Work out the finished part from the listing and answer in its coordinate system (mm). A direction names the side the tool comes from. Coordinates: 2 decimals unless noted, no trailing zeros. Loops run counter-clockwise (first coordinate to the right, second up) from the corner with the lowest first, then second, coordinate; pieces in that order, holes last. Notation, with made-up numbers: (73.5, 71) - (126.5, 71) arc R13 ccw to (126.5, 94) - close; hole circle Ø4 at (58, 68.25). An arc over 180 degrees is marked (long way). Write each question's results on one line, items separated by ' | '. Start each with the question number.
Item 1: Section D-D, the plane z = -2.4 is taken. Write down the section's boundary in (x, y).
Item 2: Consider probe 1 along X at (y, z) = (-5, 0); probe 2 along X at (y, z) = (-4.5, -0.35); probe 3 along Z at (x, y) = (-5, -3.5). Determine where each line is inside the solid, lowest interval first. Write a range as [from, to].
Item 3: Section B-B, the plane z = 0 is taken. Write down the section's boundary in (x, y).
Item 4: Section C-C, the plane y = -4.25 is taken. Write down the section's boundary in (x, z), plus the area to 3 significant figures.
Item 5: Each of these flat-tipped pins is pushed along its axis until it touches: pin 1 Ø1.9 at (x, z) = (5, 0) entering from +Y; pin 2 Ø1.1 at (x, z) = (-5, 0) entering from +Y. Where does it stop, or does it pass through?
Item 6: For a pull along X with two mould halves and no side action, classify faces 1 (the face through (-8, -4, 0)), 2 (the face through (-0.021, -1.318, -1.243)), 3 (the face through (4, -0.214, -1)), 4 (the face through (4.77, -3.954, 0.554)) as +X half, -X half, draft (parallel to the pull), parting line (faces both ways), or undercut.
Item 7: A tool of negligible diameter and unlimited length cuts with its end or side. For faces 5 (the face through (-0.021, -1.318, 1.757)), 6 (the face through (0.021, -1.318, 1.243)), 7 (the face through (0.021, -1.318, -1.757)), 8 (the face through (-5, -0.214, 1)), from which of +Z, -Z, +X, -X, +Y, -Y can it reach the whole face along a straight path? Write none if from no direction.
Item 8: Section A-A, the plane x = -5 is taken. Write down the section's boundary in (y, z).
from build123d import *

# Parameters (mm, degrees)
SKETCH_1_W               = 16
SKETCH_1_H               = 16
SKETCH_1_R               = 1.55
EXTRUDE_1_DEPTH          = 3
EXTRUDE_2_DEPTH          = 8
CUT_EXTRUDE_2_DEPTH      = 12.704699911
CUT_EXTRUDE_2_DEPTH_BACK = 12.704699911
SKETCH_8_R               = 0.6
CUT_EXTRUDE_3_DEPTH      = 12.704699911
CUT_EXTRUDE_START        = -0.2
SKETCH_10_W              = 16
SKETCH_10_H              = 6
SKETCH_10_R              = 0.6
CUT_EXTRUDE_7_DEPTH      = 0.2


with BuildPart() as part:
    # 草图1 → 凸台-拉伸1 (new, symmetric)
    with BuildSketch(Plane.XY):
        Rectangle(SKETCH_1_W, SKETCH_1_H)
        Circle(SKETCH_1_R, mode=Mode.SUBTRACT)
    extrude(amount=EXTRUDE_1_DEPTH, both=True)

    # 草图6 → 凸台-拉伸2 (add)
    with BuildSketch(Plane(origin=(0, 0, 0), x_dir=(1, 0, 0), z_dir=(0, 1, 0))):
        Polygon((-1.55, -1.743476048), (-1.55, -2.243476048), (1.55, -1.256523952), (1.55, -0.756523952), align=None)
        Polygon((-1.55, 1.256523952), (-1.55, 0.756523952), (1.55, 1.743476048), (1.55, 2.243476048), align=None)
    extrude(amount=-EXTRUDE_2_DEPTH)

    # 草图7 → 切除-拉伸2 (cut, two sides: drawn at the far end of the back side and taken through both)
    with BuildSketch(Plane.XY.offset(-CUT_EXTRUDE_2_DEPTH_BACK)):
        with BuildLine():
            Line((-8, -0.214092961), (-1.027941732, -0.214092961))
            ThreePointArc((-1.027941732, -0.214092961), (-0.107613153, 1.044470875), (1.05, 0))
            ThreePointArc((1.05, 0), (1.044470875, -0.107613153), (1.027941732, -0.214092961))
            Line((1.027941732, -0.214092961), (8, -0.214092961))
            Line((8, -0.214092961), (8, 8))
            Line((8, 8), (-8, 8))
            Line((-8, 8), (-8, -0.214092961))
        make_face()
        with BuildLine():
            Line((1.027941732, -0.214092961), (0, 0))
            Line((0, 0), (-1.027941732, -0.214092961))
            ThreePointArc((-1.027941732, -0.214092961), (0, -1.05), (1.027941732, -0.214092961))
        make_face()
        with BuildLine():
            Line((-1.027941732, -0.214092961), (0, 0))
            Line((0, 0), (1.027941732, -0.214092961))
            ThreePointArc((1.027941732, -0.214092961), (1.044470875, -0.107613153), (1.05, 0))
            ThreePointArc((1.05, 0), (-0.107613153, 1.044470875), (-1.027941732, -0.214092961))
        make_face()
    extrude(amount=CUT_EXTRUDE_2_DEPTH + CUT_EXTRUDE_2_DEPTH_BACK, mode=Mode.SUBTRACT)

    # 草图8 → 切除-拉伸3 (cut, through all)
    with BuildSketch(Plane(origin=(0, 0, 0), x_dir=(1, 0, 0), z_dir=(0, 1, 0))):
        with Locations(Location((-5, 0, 0), (0, 0, 270))):
            Circle(SKETCH_8_R)
        with Locations(Location((5, 0, 0), (0, 0, 270))):
            Circle(SKETCH_8_R)
    extrude(amount=-CUT_EXTRUDE_3_DEPTH, mode=Mode.SUBTRACT)

    # 草图10 → 切除-拉伸7 (cut)
    with BuildSketch(Plane.XZ.offset(8).offset(CUT_EXTRUDE_START)):
        Rectangle(SKETCH_10_W, SKETCH_10_H)
        with Locations(Location((-5, 0, 0), (0, 0, 180))):
            Circle(SKETCH_10_R, mode=Mode.SUBTRACT)
        with Locations((5, 0)):
            Circle(SKETCH_10_R, mode=Mode.SUBTRACT)
    extrude(amount=CUT_EXTRUDE_7_DEPTH, mode=Mode.SUBTRACT)


solid = part.part
Answer key:
1) outline: (-8, -7.8) - (8, -7.8) - (8, -0.21) - (1.54, -0.21) arc R1.55 cw to (-1.54, -0.21) - (-8, -0.21) - close
2) probe 1: x = [-8, -5.6], [-4.4, 4.4], [5.6, 8] | probe 2: x = [-8, -5.49], [-4.51, 4.51], [5.49, 8] | probe 3: z = [-3, -0.6], [0.6, 3]
3) outline: (-8, -7.8) - (-5.6, -7.8) - (-5.6, -0.21) - (-8, -0.21) - close; (-4.4, -7.8) - (4.4, -7.8) - (4.4, -0.21) - (1.54, -0.21) arc R1.55 cw to (-1.54, -0.21) - (-4.4, -0.21) - close; (5.6, -7.8) - (8, -7.8) - (8, -0.21) - (5.6, -0.21) - close
4) outline: (-8, -3) - (8, -3) - (8, 3) - (-8, 3) - close; hole circle Ø1.2 at (-5, 0); hole circle Ø1.2 at (5, 0) | area: 93.7 mm^2
5) pin 1: stops at y = -0.21 | pin 2: passes through
6) face 1: -X half | face 2: undercut | face 3: draft | face 4: undercut
7) face 5: +Z, +Y | face 6: +Y | face 7: -Z, +Y | face 8: +Z, -Z, +X, -X, +Y
8) outline: (-7.8, -3) - (-0.21, -3) - (-0.21, -0.6) - (-7.8, -0.6) - close; (-7.8, 0.6) - (-0.21, 0.6) - (-0.21, 3) - (-7.8, 3) - close
